Here's how the part is built. I have some questions about the finished solid (model axes, mm). Coordinates: 2 decimals unless noted, no trailing zeros. Write each loop counter-clockwise with the first axis right and the second up, starting at its lowest first coordinate (ties: lowest second). Pieces come first, ordered by that corner, then holes. Notation, with made-up numbers: M 59,-20 L 114,-20 A24 cw 114,-6 Z; hole C 42.25,25.25 d11. An arc over 180 degrees is marked long. Write each question's results on one line, items separated by ' | '. Start each with the question number.
from build123d import *

# Parameters (mm, degrees)
SKETCH_1_R      = 18
SKETCH_1_R_2    = 3
EXTRUDE_1_DEPTH = 2
SKETCH_2_W      = 22.533370453
SKETCH_2_H      = 20
SKETCH_2_R      = 2.5
EXTRUDE_2_DEPTH = 2
SKETCH_3_W      = 20
SKETCH_3_H      = 45
SKETCH_3_R      = 1.5
EXTRUDE_3_DEPTH = 2
FILLET_1_R      = 5
FILLET_2_R      = 8


with BuildPart() as part:
    # 草图1 → 凸台-拉伸1 (new body)
    with BuildSketch(Plane.XY):
        Circle(SKETCH_1_R)
        Circle(SKETCH_1_R_2, mode=Mode.SUBTRACT)
    extrude(amount=EXTRUDE_1_DEPTH)

    # 草图2 → 凸台-拉伸2 (add)
    # profile 1 of 2: a face of its own
    with BuildSketch(Plane.XY.offset(2)):
        with Locations((-26.233314773, 0)):
            Rectangle(SKETCH_2_W, SKETCH_2_H)
        with Locations((-30, 0)):
            Circle(SKETCH_2_R, mode=Mode.SUBTRACT)
    # profile 2 of 2: a face of its own
    with BuildSketch(Plane.XY.offset(2)):
        with Locations((26.233314773, 0)):
            Rectangle(SKETCH_2_W, SKETCH_2_H)
        with Locations((30, 0)):
            Circle(SKETCH_2_R, mode=Mode.SUBTRACT)
    extrude(amount=-EXTRUDE_2_DEPTH)

    # 草图3 → 凸台-拉伸3 (add)
    with BuildSketch(Plane.XY.offset(2)):
        with Locations((0, 32.5)):
            Rectangle(SKETCH_3_W, SKETCH_3_H)
        with Locations((-5, 50)):
            Circle(SKETCH_3_R, mode=Mode.SUBTRACT)
        with Locations((-5, 40)):
            Circle(SKETCH_3_R, mode=Mode.SUBTRACT)
        with Locations((5, 40)):
            Circle(SKETCH_3_R, mode=Mode.SUBTRACT)
        with Locations((5, 50)):
            Circle(SKETCH_3_R, mode=Mode.SUBTRACT)
    extrude(amount=-EXTRUDE_3_DEPTH)

    # 圆角1
    fillet_1_edges = [part.edges().sort_by_distance(p)[0] for p in [
        (-10, 14.966629547, 1),
        (10, 14.966629547, 1),
        (10, 55, 1),
        (-10, 55, 1),
    ]]
    fillet(fillet_1_edges, radius=FILLET_1_R)

    # 圆角2
    fillet_2_edges = [part.edges().sort_by_distance(p)[0] for p in [
        (37.5, -10, 1),
        (14.966629547, -10, 1),
        (14.966629547, 10, 1),
        (37.5, 10, 1),
        (-37.5, 10, 1),
        (-14.966629547, 10, 1),
        (-14.966629547, -10, 1),
        (-37.5, -10, 1),
    ]]
    fillet(fillet_2_edges, radius=FILLET_2_R)


solid = part.part
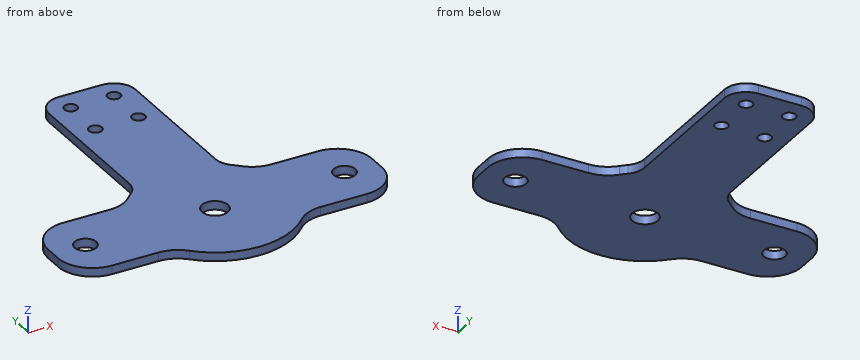
1) I want a section at C-C, the plane y = 40. Write out the boundary of the cut face in (x, z), then the cut area to 3 significant figures.
2) I want a section at D-D, the plane x = -22.5. Write out the boundary of the cut face in (y, z), then the cut area to 3 significant figures.
3) Please list where these lines run through material, in increasing order: line 1 (X direction, y = 39, z = 1.7); line 2 (Y direction, x = -30, z = 1.2); line 3 (Y direction, x = -5, z = 1.1). Write a range as [from, to].
4) I want a section at A-A, the plane x = 0. Write out the boundary of the cut face in (y, z), then the cut area to 3 significant figures.
5) I want a section at B-B, the plane z = 1.3. Give the number of separate pieces and of enclosed holes in the cut face, then the cut area to 3 significant figures.
6) For pin 1 Ø4 at (x, y) = (25, -4.5) entering from -Z; pin 2 Ø1 at (x, z) = (24, 0.5) entering from +Y; pin 3 Ø1 at (x, z) = (-24, 1) entering from -Y; pin 4 Ø2.5 at (x, y) = (5, 40) entering from -Z, each with a flat end and sliding along its axis, tell me the tip position at first contact or that it passes through.
Output:
1) outline: M -10,0 L -6.5,0 L -6.5,2 L -10,2 Z; M -3.5,0 L 3.5,0 L 3.5,2 L -3.5,2 Z; M 6.5,0 L 10,0 L 10,2 L 6.5,2 Z | area: 28.0 mm2
2) outline: M -10,0 L 10,0 L 10,2 L -10,2 Z | area: 40.0 mm2
3) line 1: x = [-10, -6.12], [-3.88, 3.88], [6.12, 10] | line 2: y = [-9.98, -2.5], [2.5, 9.98] | line 3: y = [-17.29, 38.5], [41.5, 48.5], [51.5, 55]
4) outline: M -18,0 L -3,0 L -3,2 L -18,2 Z; M 3,0 L 55,0 L 55,2 L 3,2 Z | area: 134 mm2
5) separate pieces: 1 | enclosed holes: 7 | area: 2,440 mm2
6) pin 1: stops at z = 0 | pin 2: stops at y = 10 | pin 3: stops at y = -10 | pin 4: passes through
